```python
from build123d import *

# Parameters (mm, degrees)
BOSS_EXTRUDE1_DEPTH     = 45
SKETCH2_R               = 12.5
BOSS_EXTRUDE2_DEPTH     = 3
SKETCH3_R               = 9.525
CUT_EXTRUDE1_DEPTH      = 14
SKETCH4_R               = 4
CUT_EXTRUDE2_DEPTH      = 14
SKETCH5_R               = 1.5
CUT_EXTRUDE3_DEPTH      = 14
CUT_EXTRUDE3_DEPTH_BACK = 14


with BuildPart() as part:
    # Sketch1 → Boss-Extrude1 (new body)
    with BuildSketch(Plane(origin=(0, 0, 0), x_dir=(0, 0, -1), z_dir=(1, 0, 0))):
        with BuildLine():
            Line((-14.706866163, -5.593217306), (-15.732926593, -2.774139444))
            ThreePointArc((-15.732926593, -2.774139444), (0, 0), (15.732926593, -2.774139444))
            Line((15.732926593, -2.774139444), (14.706866163, -5.593217306))
            ThreePointArc((14.706866163, -5.593217306), (0, -3), (-14.706866163, -5.593217306))
        make_face()
    extrude(amount=BOSS_EXTRUDE1_DEPTH)

    # Sketch2 → Boss-Extrude2 (add)
    with BuildSketch(Plane(origin=(0, -3, 0), x_dir=(1, 0, 0), z_dir=(0, 1, 0))):
        with Locations((22.5, 0)):
            Circle(SKETCH2_R)
    extrude(amount=-BOSS_EXTRUDE2_DEPTH)

    # Sketch3 → Cut-Extrude1 (cut)
    with BuildSketch(Plane(origin=(0, -3, 0), x_dir=(1, 0, 0), z_dir=(0, 1, 0))):
        with Locations((22.5, 0)):
            Circle(SKETCH3_R)
    extrude(amount=CUT_EXTRUDE1_DEPTH, mode=Mode.SUBTRACT)

    # Sketch4 → Cut-Extrude2 (cut)
    with BuildSketch(Plane(origin=(0, -3, 0), x_dir=(1, 0, 0), z_dir=(0, 1, 0))):
        with Locations((22.5, 0)):
            Circle(SKETCH4_R)
    extrude(amount=-CUT_EXTRUDE2_DEPTH, mode=Mode.SUBTRACT)

    # Sketch5 → Cut-Extrude3 (cut, two sides)
    with BuildSketch(Plane(origin=(0, -3, 0), x_dir=(1, 0, 0), z_dir=(0, 1, 0))) as cut_extrude3_sk:
        with Locations((6, 0)):
            Circle(SKETCH5_R)
        with Locations((39, 0)):
            Circle(SKETCH5_R)
    extrude(amount=CUT_EXTRUDE3_DEPTH, mode=Mode.SUBTRACT)
    extrude(cut_extrude3_sk.sketch, amount=-CUT_EXTRUDE3_DEPTH_BACK, mode=Mode.SUBTRACT)


solid = part.part
```
Geometry: final body of the model. Coordinates: model frame, mm. A direction names the side the tool comes from. Give positions to 0.01 mm unless a question says otherwise; leave off trailing zeros. Loops run counter-clockwise (first coordinate to the right, second up) from the corner with the lowest first, then second, coordinate; pieces in that order, holes last. Notation, with made-up numbers: (-10, -1) -> (47, -1) arc R30 ccw to (47, 22) -> close; hole circle Ø7 at (-36.5, 58.25). An arc over 180 degrees is marked (long way). Return JSON: item names as keys, results as strings.
Item 1: Section D-D, the plane y = -1.75. Output: boundary loops of the cut face in (x, z) (3 decimals).
Filled in:
{"outline": "(0, -12.567) -> (45, -12.567) -> (45, 12.567) -> (0, 12.567) -> close; hole circle Ø3 at (6, 0); hole circle Ø19.05 at (22.5, 0); hole circle Ø3 at (39, 0)"}
Item 2: Section A-A, the plane z = 0. Output: boundary loops of the cut face in (x, y) (3 decimals).
Filled in:
{"outline": "(0, -3) -> (4.5, -3) -> (4.5, 0) -> (0, 0) -> close; (7.5, -3) -> (10, -3) -> (10, -6) -> (18.5, -6) -> (18.5, -3) -> (12.975, -3) -> (12.975, 0) -> (7.5, 0) -> close; (26.5, -6) -> (35, -6) -> (35, -3) -> (37.5, -3) -> (37.5, 0) -> (32.025, 0) -> (32.025, -3) -> (26.5, -3) -> close; (40.5, -3) -> (45, -3) -> (45, 0) -> (40.5, 0) -> close"}
Item 3: Section B-B, the plane x = 22.5. Output: boundary loops of the cut face in (y, z) (3 decimals).
Filled in:
{"outline": "(-6, -12.5) -> (-4.857, -12.5) arc R43 cw to (-5.593, -14.707) -> (-2.774, -15.733) arc R46 ccw to (-0.997, -9.525) -> (-3, -9.525) -> (-3, -4) -> (-6, -4) -> close; (-6, 4) -> (-3, 4) -> (-3, 9.525) -> (-0.997, 9.525) arc R46 ccw to (-2.774, 15.733) -> (-5.593, 14.707) arc R43 cw to (-4.857, 12.5) -> (-6, 12.5) -> close"}
Item 4: Access query for faces 1 (the cylindrical face through (22.18, -4.99, 12.93)), 2 (the cylindrical face through (4.5, -1.49, -0.07)), 3 (the flat face through (27, -3, 0)). Directions: +Z, -Z, +X, -X, +Y, -Y. A direction counts if a zero-diameter tool reaches every point of the face in a straight line with its end or side. Return the directions, or none.
Filled in:
{"face 1": "-Y", "face 2": "+Y, -Y", "face 3": "+Y"}
Item 5: Line query: line 1 (X direction, y = -1.4, z = 0) (3 decimals); line 2 (X direction, y = -4.8, z = 0); line 3 (X direction, y = -3.75, z = -1.5). Output: solid intervals per line, ascending.
Filled in:
{"line 1": "0 to 4.5, 7.5 to 12.975, 32.025 to 37.5, 40.5 to 45", "line 2": "10 to 18.5, 26.5 to 35", "line 3": "10.09 to 18.79, 26.21 to 34.91"}
Item 6: Pin query (flat end, axial travel): P1, Ø4, axis at x = 39, z = 0, coming from the -Y side; P2, Ø1.5, axis at x = 30.5, y = -4, coming from the +Z side; P3, Ø1.5, axis at x = 31.5, y = -5.5, coming from the +Z side. Return the tip coordinate at first contact, or that it passes through.
Filled in:
{"P1": "y = -3.05", "P2": "z = 15.56", "P3": "z = 15.01"}
Item 7: Section C-C, the plane z = -3.5. Output: boundary loops of the cut face in (x, y), plus the area to 3 significant figures.
Filled in:
{"outline": "(0, -3.14) -> (10.5, -3.14) -> (10.5, -6) -> (20.56, -6) -> (20.56, -3) -> (13.64, -3) -> (13.64, -0.13) -> (0, -0.13) -> close; (24.44, -6) -> (34.5, -6) -> (34.5, -3.14) -> (45, -3.14) -> (45, -0.13) -> (31.36, -0.13) -> (31.36, -3) -> (24.44, -3) -> close", "area": "142 mm^2"}
